Source: three-view drawing plus pictorial views. Frame: mm from the lowest corner of the part. Coordinates: 2 decimals unless noted, no trailing zeros. Write each loop counter-clockwise with the first axis right and the second up, starting at its lowest first coordinate (ties: lowest second). Pieces come first, ordered by that corner, then holes. Notation, with made-up numbers: (72.5, -36) -> (125.5, -36) arc R18 ccw to (125.5, -15) -> close; hole circle Ø8 at (61.25, 18.5). An arc over 180 degrees is marked (long way). One line per item, written item: value.
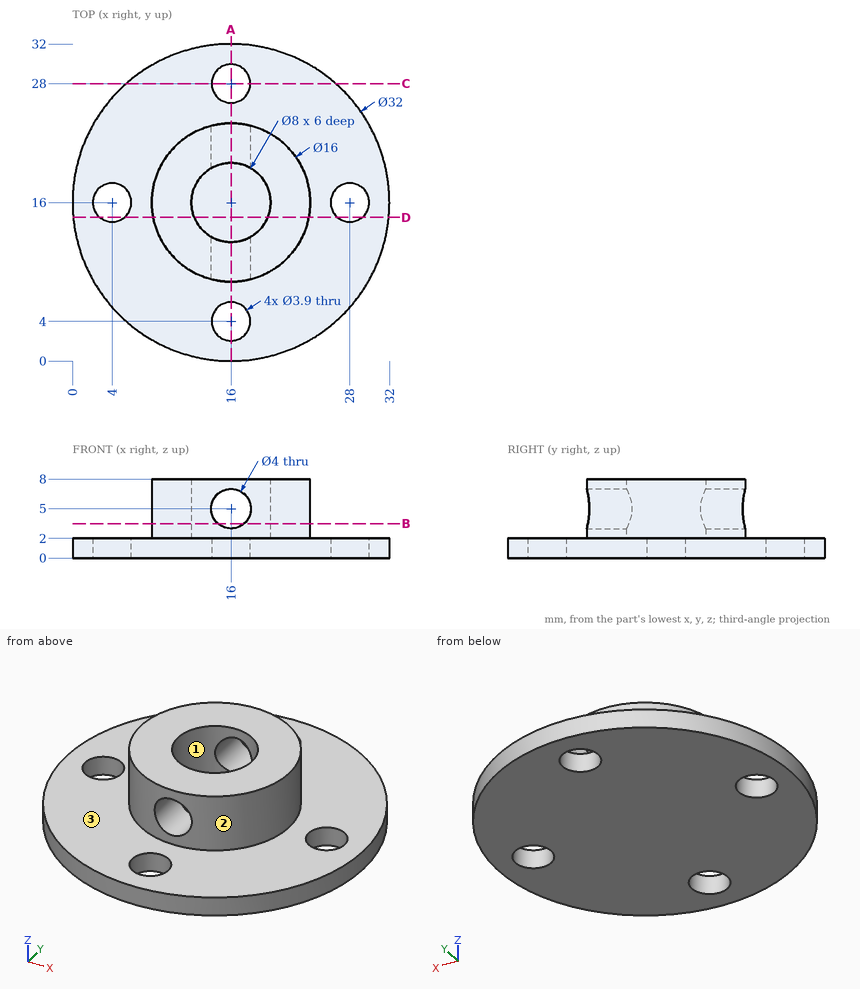
(1) Line query: line 1 (Y direction, x = 16, z = 1.3); line 2 (Z direction, x = 16, y = 10); line 3 (Z direction, x = 4, y = 14). Output: solid intervals per line, ascending. Write a range as [from, to].
Responses:
line 1: y = [0, 2.05], [5.95, 26.05], [29.95, 32]
line 2: z = [0, 3], [7, 8]
line 3: z = [0, 2]
(2) Section B-B (z = 3.5). Return the cut outline in (x, y), then the cut area to 3 significant figures.
Responses:
outline: (14.68, 8.11) -> (14.68, 12.23) arc R4 cw to (14.68, 19.77) -> (14.68, 23.89) arc R8 ccw to start; (17.32, 8.11) arc R8 ccw to (17.32, 23.89) -> (17.32, 19.77) arc R4 cw to (17.32, 12.23) -> close
area: 129 mm2
(3) Pull-direction query (X, two-part tool) for the marked faces 1, 2 and 3; classes: released by +X, released by -X, zero draft, split by the parting line, or undercut.
Responses:
face 1: undercut
face 2: split by the parting line
face 3: zero draft
(4) Section C-C (y = 28). Return the cut outline in (x, z), then the cut area to 3 significant figures.
Responses:
outline: (5.42, 0) -> (14.05, 0) -> (14.05, 2) -> (5.42, 2) -> close; (17.95, 0) -> (26.58, 0) -> (26.58, 2) -> (17.95, 2) -> close
area: 34.5 mm2
(5) Section D-D (y = 14.5). Return the cut outline in (x, z).
Responses:
outline: (0.07, 0) -> (2.75, 0) -> (2.75, 2) -> (0.07, 2) -> close; (5.25, 0) -> (26.75, 0) -> (26.75, 2) -> (23.86, 2) -> (23.86, 8) -> (19.71, 8) -> (19.71, 2) -> (12.29, 2) -> (12.29, 8) -> (8.14, 8) -> (8.14, 2) -> (5.25, 2) -> close; (29.25, 0) -> (31.93, 0) -> (31.93, 2) -> (29.25, 2) -> close
(6) First-contact query: pin 1 (2.5 mm diameter, centred on x = 16, y = 28, fed in from -Z) (3 decimals); pin 2 (4.5 mm diameter, centred on x = 16, z = 5, fed in from -Y); pin 3 (4 mm diameter, centred on x = 16, y = 15.5, fed in from +Z). Flat tips, straight axial feed; report the tip coordinate or a pass-through.
Responses:
pin 1: passes through
pin 2: stops at y = 8
pin 3: stops at z = 2
(7) Section A-A (x = 16). Return the cut outline in (y, z), then the cut area to 3 significant figures.
Responses:
outline: (0, 0) -> (2.05, 0) -> (2.05, 2) -> (0, 2) -> close; (5.95, 0) -> (26.05, 0) -> (26.05, 2) -> (24, 2) -> (24, 3) -> (20, 3) -> (20, 2) -> (12, 2) -> (12, 3) -> (8, 3) -> (8, 2) -> (5.95, 2) -> close; (8, 7) -> (12, 7) -> (12, 8) -> (8, 8) -> close; (20, 7) -> (24, 7) -> (24, 8) -> (20, 8) -> close; (29.95, 0) -> (32, 0) -> (32, 2) -> (29.95, 2) -> close
area: 64.4 mm2
